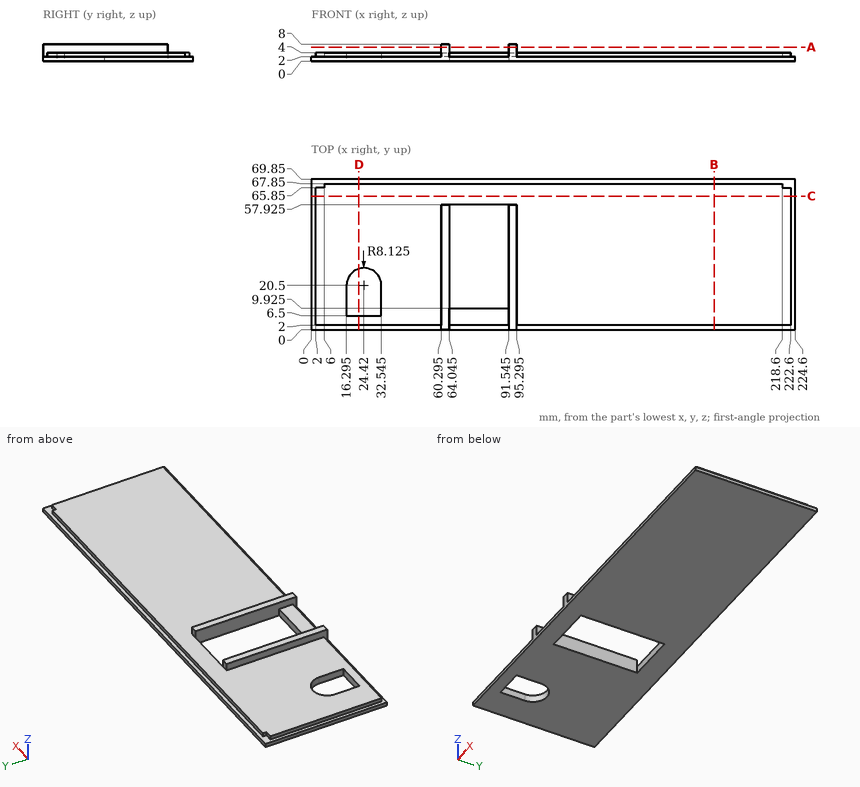
Verification items for this drawing (mm, ordinates from the low corner). Round coordinates to 2 decimals unless told otherwise and drop trailing zeros. Order: outer loops, then holes, each group sorted by start corner. A loop starts at its lowest first (then second) coordinate and runs counter-clockwise, first axis right, second up.
1) Material ranges on line 1 (X direction, y = 12, z = 3.5) (1 decimal); line 2 (X direction, y = 45, z = 3.75) (1 decimal); line 3 (X direction, y = 37, z = 1.5) (1 decimal), recorded low to high.
Geometry says:
line 1: x = 2 to 16.3, 32.5 to 64, 91.5 to 222.6
line 2: x = 2 to 64, 91.5 to 222.6
line 3: x = 0 to 64, 91.5 to 224.6
2) Cross-section at A-A, the plane z = 6.5. Record the cut outline in (x, y) (1 decimal).
Geometry says:
outline: (60.3, 0) - (64, 0) - (64, 57.9) - (60.3, 57.9) - close; (91.5, 0) - (95.3, 0) - (95.3, 57.9) - (91.5, 57.9) - close
3) Cross-section at C-C, the plane y = 62. Record the cut outline in (x, z).
Geometry says:
outline: (0, 0) - (224.6, 0) - (224.6, 2) - (222.6, 2) - (222.6, 4) - (2, 4) - (2, 2) - (0, 2) - close
4) Cross-section at D-D, the plane x = 22. Record the cut outline in (y, z).
Geometry says:
outline: (0, 0) - (6.5, 0) - (6.5, 4) - (2, 4) - (2, 2) - (0, 2) - close; (28.26, 0) - (69.85, 0) - (69.85, 2) - (67.85, 2) - (67.85, 4) - (28.26, 4) - close
5) Depth check by flat-ended pin: pin 1 (1 mm diameter, centred on y = 67, z = 3, fed in from +X); pin 2 (1.1 mm diameter, centred on x = 62.5, z = 6.5, fed in from +Y) (3 decimals); pin 3 (0.6 mm diameter, centred on x = 4, z = 3.5, fed in from +Y); pin 4 (5 mm diameter, centred on x = 110, y = 12, fed in from -Z). Enter the tip coordinate at first touch or a pass-through.
Geometry says:
pin 1: stops at x = 218.6
pin 2: stops at y = 57.925
pin 3: stops at y = 65.85
pin 4: stops at z = 0
6) Cross-section at B-B, the plane x = 187. Record the cut outline in (y, z), plus the area to 3 significant figures.
Geometry says:
outline: (0, 0) - (69.85, 0) - (69.85, 2) - (67.85, 2) - (67.85, 4) - (2, 4) - (2, 2) - (0, 2) - close
area: 271 mm2
